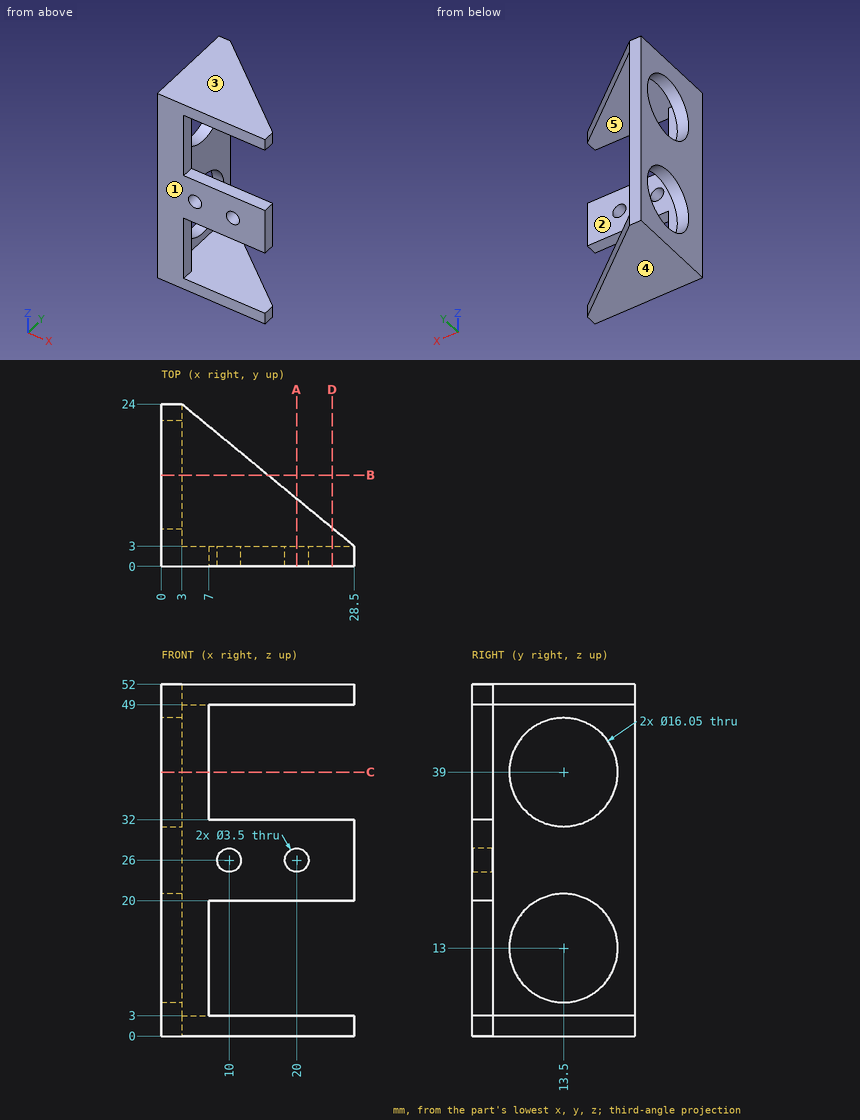
Could you check a few things on this drawing? It's one solid part, dimensions in mm from its lowest x, y, z. A direction names the side the tool comes from. Round coordinates to 2 decimals unless told otherwise and drop trailing zeros. Loops run counter-clockwise (first coordinate to the right, second up) from the corner with the lowest first, then second, coordinate; pieces in that order, holes last.
Q1. I want a section at D-D (x = 25.25). Write out the boundary of the cut face in (y, z), and give its area (3 significant figures).
Q2. Please list where these lines run through material, in increasing order: L1, parallel to X at y = 0.8, z = 26; L2, parallel to Z at x = 21.75, y = 3.5; L3, parallel to Y at x = 0.85, z = 13 (3 decimals).
Q3. On a 3-axis mill with a long thin cutter (end or side, diameter ignored), from which of +Z, -Z, +X, -X, +Y, -Y can I reach the whole of each face in a straight line? I mean the marked faces 4 and 5. Say none if no direction works.
Q4. I want a section at A-A (x = 20). Write out the boundary of the cut face in (y, z), and give its area (3 significant figures).
Q5. I want a section at B-B (y = 13.5). Write out the boundary of the cut face in (x, z) (3 decimals).
Q6. For P1, Ø10, axis at y = 11, z = 26.5, coming from the +X side; P2, Ø3.5, axis at y = 1.5, z = 42.5, coming from the +X side; P3, Ø9.5, axis at y = 13.5, z = 39, coming from the -X side; P4, Ø1, axis at x = 16.5, z = 27, coming from the +Y side, each with a flat end and sliding along its axis, tell me the tip position at first contact or that it passes through.
Q7. I want a section at C-C (z = 39). Write out the boundary of the cut face in (x, y) (3 decimals).
Q8. Thinking about a two-plate mould opening in Z: for the marked faces 1, 2 and 3, which applies, pulls with the +Z half, pulls with the -Z half, needs draft (parallel to the pull), parting line crosses it, or undercut?
Answer below:
1. outline: (0, 0) - (5.68, 0) - (5.68, 3) - (0, 3) - close; (0, 20) - (3, 20) - (3, 32) - (0, 32) - close; (0, 49) - (5.68, 49) - (5.68, 52) - (0, 52) - close
1. area: 70.1 mm2
2. L1: x = 0 to 8.25, 11.75 to 18.25, 21.75 to 28.5
2. L2: z = 0 to 3, 49 to 52
2. L3: y = 0 to 5.475, 21.525 to 24
3. face 4: -Z, +X, -X, +Y, -Y
3. face 5: +X, +Y
4. outline: (0, 0) - (10, 0) - (10, 3) - (0, 3) - close; (0, 20) - (3, 20) - (3, 24.25) - (0, 24.25) - close; (0, 27.75) - (3, 27.75) - (3, 32) - (0, 32) - close; (0, 49) - (10, 49) - (10, 52) - (0, 52) - close
4. area: 85.5 mm2
5. outline: (0, 0) - (15.75, 0) - (15.75, 3) - (3, 3) - (3, 4.975) - (0, 4.975) - close; (0, 21.025) - (3, 21.025) - (3, 30.975) - (0, 30.975) - close; (0, 47.025) - (3, 47.025) - (3, 49) - (15.75, 49) - (15.75, 52) - (0, 52) - close
6. P1: stops at x = 3
6. P2: stops at x = 7
6. P3: passes through
6. P4: stops at y = 3
7. outline: (0, 0) - (7, 0) - (7, 3) - (3, 3) - (3, 5.475) - (0, 5.475) - close; (0, 21.525) - (3, 21.525) - (3, 24) - (0, 24) - close
8. face 1: needs draft
8. face 2: undercut
8. face 3: pulls with the +Z half
